from build123d import *

# Parameters (mm, degrees)
F3_DEPTH = 5


with BuildPart() as f1:
    # F0 (on Front) → F1 (revolve)
    with BuildSketch(Plane.XZ):
        with BuildLine():
            Line((-32.54427, -50.761096), (0, -50.761096))
            Line((0, -50.761096), (0, 21.635026))
            Line((0, 21.635026), (-16.303314, 21.635026))
            Line((-16.303314, 21.635026), (-16.303314, 12.826373))
            Line((-16.303314, 12.826373), (-11.073175, 0))
            Line((-11.073175, 0), (-14.926962, -7.54364))
            Line((-14.926962, -7.54364), (-14.926962, -35.345953))
            Line((-14.926962, -35.345953), (-29.548365, -41.742818))
            ThreePointArc((-29.548365, -41.742818), (-31.728794, -43.586861), (-32.54427, -46.323604))
            Line((-32.54427, -46.323604), (-32.54427, -50.761096))
        make_face()
    revolve(axis=Axis((0, 0, -14.563035), (0, 0, -1)))

    # F2 (on Front) → F3 (join)
    with BuildSketch(Plane.XZ):
        Polygon((-2.04105, 21.477198), (1.649017, 21.728793), (1.649017, 25.25113), (5.506815, 25.334995), (5.506815, 26.592974), (1.732882, 26.676839), (1.816748, 29.612118), (-1.453994, 29.695984), (-1.621724, 26.592974), (-4.808601, 26.509108), (-4.724736, 25.502726), (-2.04105, 25.167266), align=None)
    extrude(amount=F3_DEPTH)

    # F4: F1 across face


with BuildPart() as f1_1:
    add(f1.part)
    add(f1.part.mirror(Plane(origin=(0.130619, 0, 25.64342), x_dir=(1, 0, 0), z_dir=(0, 1, 0))))


solid = f1_1.part
Model file for the job. Use its own axes, mm. A direction names the side the tool comes from. Give positions to 0.01 mm unless a question says otherwise; leave off trailing zeros. Write each loop counter-clockwise with the first axis right and the second up, starting at its lowest first coordinate (ties: lowest second). Pieces come first, ordered by that corner, then holes. Notation, with made-up numbers: (83.25, -35) - (126.25, -35) arc R8 cw to (126.25, -29) - close; hole circle Ø3 at (-29, 23). An arc over 180 degrees is marked (long way). Answer as CSV lines item,"result".
1. Pin check, flat tips, straight feed: pin 1 (4 mm diameter, centred on y = 1.5, z = 23.5, fed in from -X); pin 2 (6.5 mm diameter, centred on x = -1, z = 26, fed in from -Y); pin 3 (0.6 mm diameter, centred on y = 1.5, z = 26, fed in from +X). Stop position of each tip, or through.
Responses:
pin 1,"stops at x = -16.28"
pin 2,"stops at y = -5"
pin 3,"stops at x = 5.51"
2. Two-plate mould, pull along Z, no slides. Class faces 1 (the face through (1.649, 0, 23)), 2 (the face through (-1.537, -0.07, 28.166)), 3 (the face through (0, -5, 26)): +Z half, -Z half, draft (parallel to the pull), parting line (faces both ways), or undercut.
Responses:
face 1,"undercut"
face 2,"+Z half"
face 3,"draft"
3. Band-saw the part on A-A (z = 20.5). Write the cut outline in (x, y).
Responses:
outline,"circle Ø32.61 at (0, 0)"
4. 3-axis set-ups, long thin cutter, end or side, ignore diameter. For faces 4 (the face through (-2.041, 0, 23)), 5 (the face through (12.94, -9.92, 17.17)), 6 (the face through (2.453, -11.045, -0.472)): which of +Z, -Z, +X, -X, +Y, -Y reach the whole face in a straight line?
Responses:
face 4,"-X, +Y, -Y"
face 5,"+Z"
face 6,"none"
5. Drill centre lines: L1, parallel to Z at x = -5, y = -13; L2, parallel to Z at x = -4.5, y = 6; L3, parallel to Z at x = -0.5, y = 24. Where is each one in solid material? Low to high. Write a range as [from, to].
Responses:
L1,"z = [-50.76, -5.59], [7, 21.64]"
L2,"z = [-50.76, 21.64]"
L3,"z = [-50.76, -39.32]"
6. Band-saw the part on C-C (z = -30.5). Write the cut outline in (x, y), and give its area (3 significant figures).
Responses:
outline,"circle Ø29.85 at (0, 0)"
area,"700 mm2"
